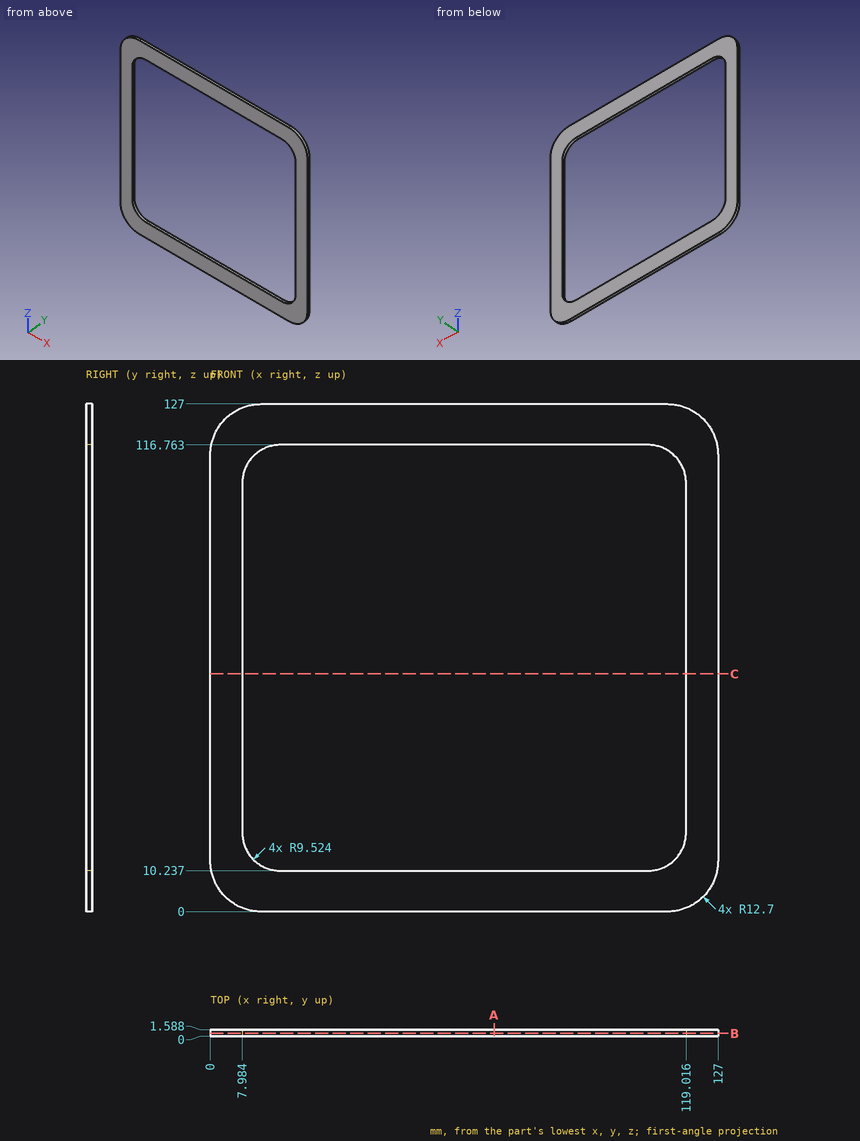
Print and shaded views of the part. All mm, measured from the part's lowest x, y and z. Give positions to 0.01 mm unless a question says otherwise; leave off trailing zeros. Write each loop counter-clockwise with the first axis right and the second up, starting at its lowest first coordinate (ties: lowest second). Pieces come first, ordered by that corner, then holes. Notation, with made-up numbers: (-32.75, 39.5) - (-19.75, 39.5) arc R29 ccw to (-19.75, 68.5) - close; hole circle Ø7 at (81, -40). An arc over 180 degrees is marked (long way). One line per question, with ' | ' between items. Start each with the question number.
(1) Slice it at A-A on x = 71. Write the cut outline in (y, z).
(2) Wall check: line 1 along X through (y, z) = (1.15, 91) (1 decimal); line 2 along Z through (x, y) = (101.5, 0.4); line 3 along Z through (x, y) = (12, 0.5). Give the ranges that are in metal, low to high. Write a range as from..to.
(3) Slice it at C-C on z = 59.5. Write the cut outline in (x, y) (1 decimal).
(4) Slice it at B-B on y = 0.65. Write the cut outline in (x, z) (1 decimal), plus the area to 3 significant figures.
Results below:
1) outline: (0, 0) - (1.59, 0) - (1.59, 10.24) - (0, 10.24) - close; (0, 116.76) - (1.59, 116.76) - (1.59, 127) - (0, 127) - close
2) line 1: 0..8, 119..127 | line 2: 0..10.24, 116.76..127 | line 3: 0.02..11.99, 115.01..126.98
3) outline: (0, 0) - (8, 0) - (8, 1.6) - (0, 1.6) - close; (119, 0) - (127, 0) - (127, 1.6) - (119, 1.6) - close
4) outline: (0, 12.7) arc R12.7 ccw to (12.7, 0) - (114.3, 0) arc R12.7 ccw to (127, 12.7) - (127, 114.3) arc R12.7 ccw to (114.3, 127) - (12.7, 127) arc R12.7 ccw to (0, 114.3) - close; hole (8, 19.8) arc R9.5 ccw to (17.5, 10.2) - (109.5, 10.2) arc R9.5 ccw to (119, 19.8) - (119, 107.2) arc R9.5 ccw to (109.5, 116.8) - (17.5, 116.8) arc R9.5 ccw to (8, 107.2) - close | area: 4,240 mm^2
